Geometry check sheet. Reference: the model listing, model coordinates, mm. Round coordinates to 2 decimals unless told otherwise and drop trailing zeros. Write each loop counter-clockwise with the first axis right and the second up, starting at its lowest first coordinate (ties: lowest second). Pieces come first, ordered by that corner, then holes. Notation, with made-up numbers: M 27.5,8.25 L 69.5,8.25 A22 ccw 69.5,39.25 Z; hole C -10,47.25 d6. An arc over 180 degrees is marked long. Use a Markdown table: item, result.
```python
from build123d import *

# Parameters (mm, degrees)
BOSS_EXTRUDE1_DEPTH = 3


with BuildPart() as part:
    # Sketch1 → Boss-Extrude1 (new body)
    with BuildSketch(Plane.XY):
        with BuildLine():
            Line((1213.574821367, 135), (1242.574821367, 135))
            ThreePointArc((1242.574821367, 135), (1248.231675617, 137.343145751), (1250.574821367, 143))
            Line((1250.574821367, 143), (1250.574821367, 172))
            ThreePointArc((1250.574821367, 172), (1248.231675617, 177.656854249), (1242.574821367, 180))
            Line((1242.574821367, 180), (1213.574821367, 180))
            ThreePointArc((1213.574821367, 180), (1207.917967118, 177.656854249), (1205.574821367, 172))
            Line((1205.574821367, 172), (1205.574821367, 143))
            ThreePointArc((1205.574821367, 143), (1207.917967118, 137.343145751), (1213.574821367, 135))
        make_face()
    extrude(amount=-BOSS_EXTRUDE1_DEPTH)


solid = part.part
```
Item 1: Cross-section at A-A, the plane z = -2.25. Record the cut outline in (x, y), and give its area (3 significant figures).
Outcome:
| item | result |
|---|---|
| outline | M 1205.57,143 A8 ccw 1213.57,135 L 1242.57,135 A8 ccw 1250.57,143 L 1250.57,172 A8 ccw 1242.57,180 L 1213.57,180 A8 ccw 1205.57,172 Z |
| area | 1,970 mm2 |
Item 2: Cross-section at C-C, the plane y = 138. Record the cut outline in (x, z).
Outcome:
| item | result |
|---|---|
| outline | M 1207.33,-3 L 1248.82,-3 L 1248.82,0 L 1207.33,0 Z |
Item 3: Cross-section at B-B, the plane y = 175. Record the cut outline in (x, z).
Outcome:
| item | result |
|---|---|
| outline | M 1206.16,-3 L 1249.99,-3 L 1249.99,0 L 1206.16,0 Z |
Item 4: Material ranges on line 1 along X through (y, z) = (140, -1); line 2 along Y through (x, z) = (1209.5, -2.65); line 3 along X through (y, z) = (173, -0.3), recorded low to high. Write a range as from..to.
Outcome:
| item | result |
|---|---|
| line 1 | x = 1206.16..1249.99 |
| line 2 | y = 136.12..178.88 |
| line 3 | x = 1205.64..1250.51 |
